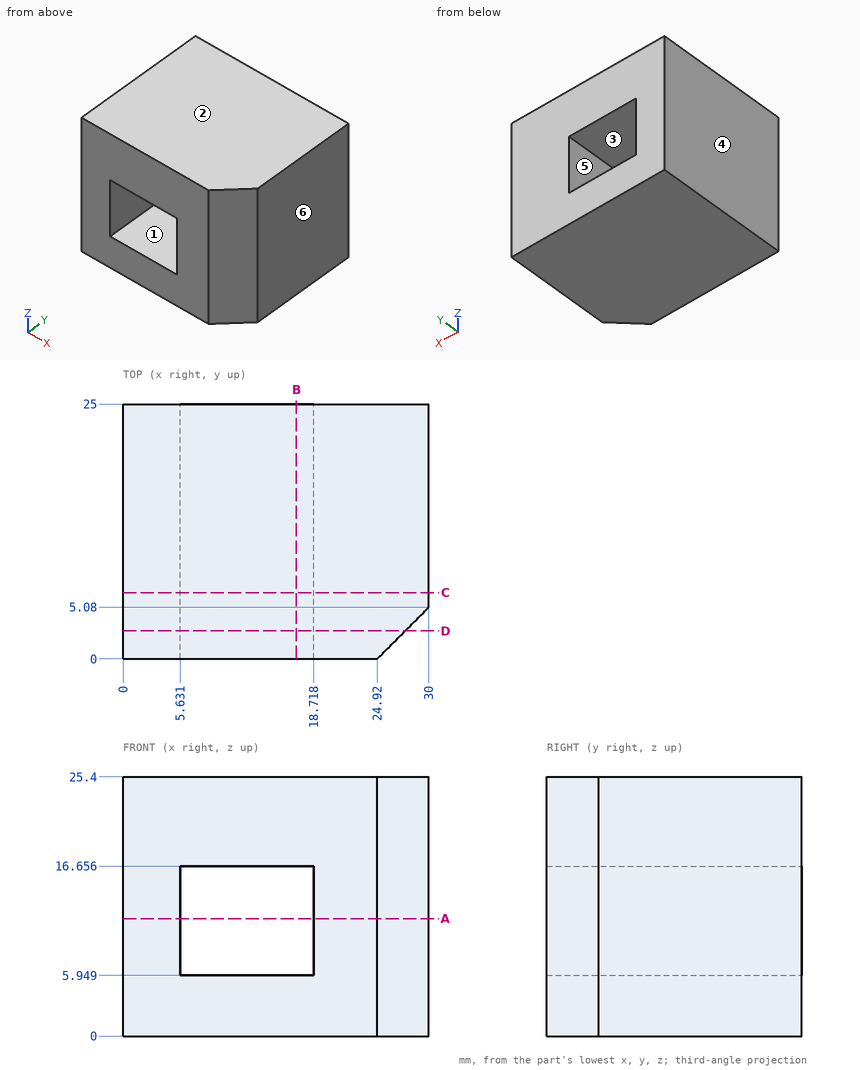
Verification items for this drawing (mm, ordinates from the low corner). A direction names the side the tool comes from. Give positions to 0.01 mm unless a question says otherwise; leave off trailing zeros. Loops run counter-clockwise (first coordinate to the right, second up) from the corner with the lowest first, then second, coordinate; pieces in that order, holes last. Notation, with made-up numbers: M -12,-19 L 5,-19 A28 cw 5,19 Z; hole C 58,45 d5. An arc over 180 degrees is marked long. Answer as a JSON object with one key per item and string values. Group by question number.
Q1. Material ranges on line 1 along Z through (x, y) = (13.5, 2.5); line 2 along X through (y, z) = (10.25, 11); line 3 along Y through (x, z) = (27, 22.25), recorded low to high. Write a range as [from, to].
Q2. Release check for a two-part mould opening along X. For the marked faces 1, 2, 3 and 4 record: released by +X, released by -X, zero draft, split by the parting line, or undercut.
Q3. Cross-section at A-A on z = 11.5. Record the cut outline in (x, y).
Q4. Cross-section at D-D on y = 2.75. Record the cut outline in (x, z).
Q5. Cross-section at C-C on y = 6.5. Record the cut outline in (x, z).
Q6. Go/stop test with a flat-tipped pin: P1, Ø10, axis at x = 21, y = 21.5, coming from the -Z side. Record where the tip stops, or that it passes through.
Q7. Access from +Z, -Z, +X, -X, +Y, -Y to the whole of each face (thin tool, end or side, straight path). Record for the marked faces 5 and 6.
Q8. Cross-section at B-B on x = 17. Record the cut outline in (y, z).
Evaluation:
{
 "1": {"line 1": "z = [0, 5.95], [16.66, 25.4]", "line 2": "x = [0, 5.63], [18.72, 30]", "line 3": "y = [2.08, 25]"},
 "2": {"face 1": "undercut", "face 2": "zero draft", "face 3": "undercut", "face 4": "released by -X"},
 "3": {"outline": "M 0,0 L 5.63,0 L 5.63,25 L 0,25 Z; M 18.72,0 L 24.92,0 L 30,5.08 L 30,25 L 18.72,25 Z"},
 "4": {"outline": "M 0,0 L 27.67,0 L 27.67,25.4 L 0,25.4 Z; hole M 5.63,5.95 L 18.72,5.95 L 18.72,16.66 L 5.63,16.66 Z"},
 "5": {"outline": "M 0,0 L 30,0 L 30,25.4 L 0,25.4 Z; hole M 5.63,5.95 L 18.72,5.95 L 18.72,16.66 L 5.63,16.66 Z"},
 "6": {"P1": "stops at z = 0"},
 "7": {"face 5": "+Y, -Y", "face 6": "+Z, -Z, +X, +Y, -Y"},
 "8": {"outline": "M 0,0 L 25,0 L 25,5.95 L 0,5.95 Z; M 0,16.66 L 25,16.66 L 25,25.4 L 0,25.4 Z"}
}
